```python
from build123d import *

# Parameters (mm, degrees)
F0_W     = 48.470514
F0_H     = 50.374654
F0_R     = 16.5
F1_DEPTH = 75
F2_DEPTH = 60
F3_R     = 5
F4_R     = 5


with BuildPart() as f1:
    # F0 (on Top) → F1 (new body)
    with BuildSketch(Plane.XY):
        with Locations((-0.40803, 0.136011)):
            Rectangle(F0_W, F0_H)
        Circle(F0_R, mode=Mode.SUBTRACT)
    extrude(amount=F1_DEPTH)

    # F0 (on Top) → F2 (join)
    with BuildSketch(Plane.XY):
        Circle(F0_R)
    extrude(amount=F2_DEPTH)

    # F3
    f3_edges = [f1.edges().sort_by_distance(p)[0] for p in [
        (23.827227, 25.323338, 37.5),
        (-24.643287, 25.323338, 37.5),
        (23.827227, -25.051316, 37.5),
        (-24.643287, -25.051316, 37.5),
    ]]
    fillet(f3_edges, radius=F3_R)

    # F4
    f4_edges = [f1.edges().sort_by_distance(p)[0] for p in [
        (-0.40803, 25.323338, 75),
        (23.827227, 0.136011, 75),
        (-0.40803, -25.051316, 75),
        (-24.643287, 0.136011, 75),
    ]]
    fillet(f4_edges, radius=F4_R)


solid = f1.part
```
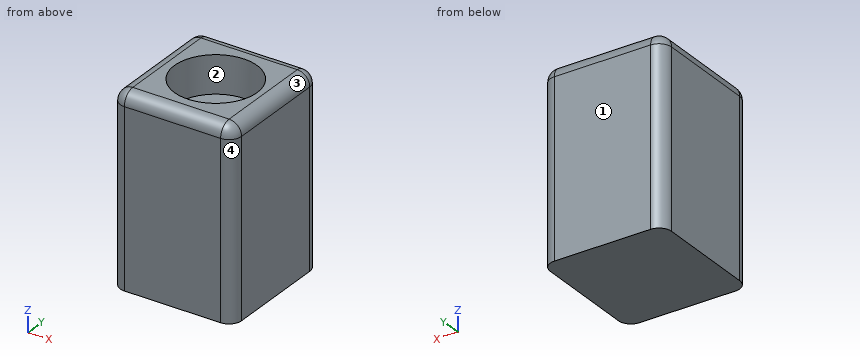
Here's how the part is built. I have some questions about the finished solid (model axes, mm). Face numbers are marked on the shaded views. Give positions to 0.01 mm unless a question says otherwise; leave off trailing zeros. Loops run counter-clockwise (first coordinate to the right, second up) from the corner with the lowest first, then second, coordinate; pieces in that order, holes last. Notation, with made-up numbers: (46.5, 46.5) -> (73.5, 46.5) arc R34 cw to (73.5, 79.5) -> close; hole circle Ø7 at (-31, 79.25). An arc over 180 degrees is marked (long way). Use one line per item in the form item = value. Start each with the question number.
1) Thinking about a two-plate mould opening in Y: for the marked faces 1, 2, 3 and 4, which applies, +Y half, -Y half, draft (parallel to the pull), parting line (faces both ways), or undercut?
2) Imagine slicing it at A-A (y = 0). Please give me the cut outline in (x, z).
3) Please list where these lines run through material, in increasing order: line 1 along Y through (x, z) = (0, 68); line 2 along Z through (x, y) = (5, 11.5); line 3 along Y through (x, z) = (-13.5, 64).
4) Imagine slicing it at B-B (x = 0). Please give me the cut outline in (y, z).
5) Imagine slicing it at C-C (x = 21.5). Please give me the cut outline in (y, z), then the cut area to 3 significant figures.
Check values:
q1.face_1 = +Y half
q1.face_2 = undercut
q1.face_3 = draft
q1.face_4 = -Y half
q2.outline = (-24.64, 0) -> (23.83, 0) -> (23.83, 70) arc R5 ccw to (18.83, 75) -> (16.5, 75) -> (16.5, 60) -> (-16.5, 60) -> (-16.5, 75) -> (-19.64, 75) arc R5 ccw to (-24.64, 70) -> close
q3.line_1 = -25.05 to -16.5, 16.5 to 25.32
q3.line_2 = 0 to 60
q3.line_3 = -25.05 to -9.49, 9.49 to 25.32
q4.outline = (-25.05, 0) -> (25.32, 0) -> (25.32, 70) arc R5 ccw to (20.32, 75) -> (16.5, 75) -> (16.5, 60) -> (-16.5, 60) -> (-16.5, 75) -> (-20.05, 75) arc R5 ccw to (-25.05, 70) -> close
q5.outline = (-24.28, 0) -> (24.55, 0) -> (24.55, 70) arc R4.23 ccw to (20.32, 74.23) -> (-20.05, 74.23) arc R4.23 ccw to (-24.28, 70) -> close
q5.area = 3,620 mm^2
